```python
from build123d import *

# Parameters (mm, degrees)
F1_DEPTH = 50.8
F3_DEPTH = 50.8
F5_DEPTH = 50.8


with BuildPart() as f1:
    # F0 (on Top) → F1 (new body)
    with BuildSketch(Plane.XY):
        Polygon((-87.056688, 106.687943), (-87.056688, -45.712057), (90.739539, -44.553774), (90.739539, 106.687943), align=None)
    extrude(amount=F1_DEPTH)

    # F2 (on face) → F3 (join)
    with BuildSketch(Plane(origin=(0, 0, 0), x_dir=(1, 0, 0), z_dir=(0, 0, -1))):
        Polygon((-36.256688, 45.381112), (-87.056688, 45.712057), (-87.056688, -30.487943), (-36.256688, -30.487943), align=None)
    extrude(amount=F3_DEPTH)

    # F4 (on face) → F5 (join)
    with BuildSketch(Plane(origin=(0, 0, 0), x_dir=(1, 0, 0), z_dir=(0, 0, -1))):
        Polygon((90.739539, 44.553774), (39.939539, 44.884719), (39.939539, -31.315281), (90.739539, -31.315281), align=None)
    extrude(amount=F5_DEPTH)


solid = f1.part
```
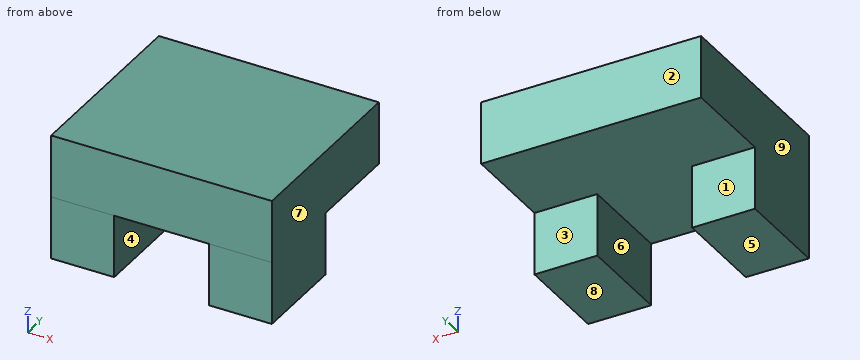
Geometry check sheet. Reference: the model listing, model coordinates, mm. Face numbers are marked on the shaded views. A direction names the side the tool comes from. Coordinates: 2 decimals unless noted, no trailing zeros. Loops run counter-clockwise (first coordinate to the right, second up) from the corner with the lowest first, then second, coordinate; pieces in that order, holes last. Notation, with made-up numbers: (84.25, 20) - (106.25, 20) arc R13 ccw to (106.25, 35) - close; hole circle Ø7 at (66, 52.5). An arc over 180 degrees is marked (long way). One line per item, written item: value. Start each with the question number.
(1) Cross-section at D-D on x = 62.5. Enter the section's corners in (y, z).
(2) Cross-section at A-A on z = -15.5. Enter the section's corners in (x, y).
(3) Material ranges on line 1 (X direction, y = 24.5, z = -25.5); line 2 (Y direction, x = -38.5, z = -32); line 3 (Z direction, x = -72, y = 80), recorded low to high. Write a range as [from, to].
(4) Depth check by flat-ended pin: P1, Ø2, axis at x = 58, z = -16, coming from the +Y side; P2, Ø3, axis at x = -66.5, y = 70, coming from the -Z side; P3, Ø8, axis at x = 50, z = -22.5, coming from the -Y side. Enter the tip coordinate at first touch or a pass-through.
(5) Mould release check, pull along X, two halves, no side actions. Record for the marked faces 6, 7, 8 and 9: released by +X, released by -X, zero draft, split by the parting line, or undercut.
(6) Cross-section at C-C on x = -48.5. Enter the section's corners in (y, z).
(7) Tool access check on the marked faces 1, 2, 3, 4 and 5. Record the directions out of +Z, -Z, +X, -X, +Y, -Y that give a thin tool (end or side, any length) a straight path to the whole face; none if there is none.
(8) Cross-section at B-B on y = 24.5. Enter the section's corners in (x, z).
Results below:
1. outline: (-44.74, -50.8) - (31.32, -50.8) - (31.32, 0) - (106.69, 0) - (106.69, 50.8) - (-44.74, 50.8) - close
2. outline: (-87.06, -45.71) - (-36.26, -45.38) - (-36.26, 30.49) - (-87.06, 30.49) - close; (39.94, -44.88) - (90.74, -44.55) - (90.74, 31.32) - (39.94, 31.32) - close
3. line 1: x = [-87.06, -36.26], [39.94, 90.74]
3. line 2: y = [-45.4, 30.49]
3. line 3: z = [0, 50.8]
4. P1: stops at y = 31.32
4. P2: stops at z = 0
4. P3: stops at y = -44.85
5. face 6: undercut
5. face 7: released by +X
5. face 8: zero draft
5. face 9: released by -X
6. outline: (-45.46, -50.8) - (30.49, -50.8) - (30.49, 0) - (106.69, 0) - (106.69, 50.8) - (-45.46, 50.8) - close
7. face 1: -Z, -X, +Y
7. face 2: +Z, -Z, +X, -X, +Y
7. face 3: -Z, +X, -X, +Y
7. face 4: -Z, +Y, -Y
7. face 5: -Z, +X, -X, +Y, -Y
8. outline: (-87.06, -50.8) - (-36.26, -50.8) - (-36.26, 0) - (39.94, 0) - (39.94, -50.8) - (90.74, -50.8) - (90.74, 50.8) - (-87.06, 50.8) - close
